Build history of the part. All positions in model axes, mm. A direction names the side the tool comes from. Give positions to 0.01 mm unless a question says otherwise; leave off trailing zeros. Loops run counter-clockwise (first coordinate to the right, second up) from the corner with the lowest first, then second, coordinate; pieces in that order, holes last. Notation, with made-up numbers: (40.5, 79) -> (82.5, 79) arc R24 ccw to (82.5, 97) -> close; hole circle Ø8 at (-6.75, -26). An arc over 180 degrees is marked (long way). Answer as a JSON object with one key per item and string values. Group by question number.
Q1. Band-saw the part on A-A, the plane y = 6. Write the cut outline in (x, z) (1 decimal).
Q2. Wall check: probe 1 along X at (y, z) = (19, -53) (1 decimal); probe 2 along Y at (x, z) = (683.5, -31.5). Give the ranges that are in metal, low to high. Write a range as from..to.
Q3. Drop flat-ended pins along their axis: pin 1 (9.5 mm diameter, centred on y = 8, z = -32, fed in from -X); pin 2 (1.5 mm diameter, centred on x = 700.5, z = -28.5, fed in from -Y). Give the stop position or say it passes through.
Q4. Band-saw the part on C-C, the plane x = 724.5. Write the cut outline in (y, z), plus the area to 3 significant figures.
Q5. Two-plate mould, pull along X, no slides. Class faces 1 (the flat face through (738.188, 9, -44)), 2 (the flat face through (790.575, 19, -44)), 3 (the flat face through (392, 0, -45)): pulls with the +X half, pulls with the -X half, needs draft (parallel to the pull), parting line crosses it, or undercut.
Q6. Tool access for faces 4 (the flat face through (96, 19.05, -44)), 5 (the flat face through (390, 38.1, -45)): list every direction of +Z, -Z, +X, -X, +Y, -Y with a clear straight run to the whole face (end or side of a thin tool).
from build123d import *

# Parameters (mm, degrees)
SKETCH1_W           = 790.575
SKETCH1_H           = 88.9
BOSS_EXTRUDE1_DEPTH = 38.1
SKETCH2_W           = 88.9
SKETCH2_H           = 19.05
CUT_EXTRUDE1_DEPTH  = 89.9


with BuildPart() as part:
    # Sketch1 → Boss-Extrude1 (new body)
    with BuildSketch(Plane(origin=(0, 0, 0), x_dir=(1, 0, 0), z_dir=(0, 1, 0))):
        with Locations((395.2875, 44.45)):
            Rectangle(SKETCH1_W, SKETCH1_H)
    extrude(amount=BOSS_EXTRUDE1_DEPTH)

    # Sketch2 → Cut-Extrude1 (cut, through all)
    with BuildSketch(Plane.XY):
        with Locations((693.7375, 9.525)):
            Rectangle(SKETCH2_W, SKETCH2_H)
        with Locations((96.8502, 9.525)):
            Rectangle(SKETCH2_W, SKETCH2_H)
    extrude(amount=-CUT_EXTRUDE1_DEPTH, mode=Mode.SUBTRACT)


solid = part.part
Worked answers:
{
 "1": {"outline": "(0, -88.9) -> (52.4, -88.9) -> (52.4, 0) -> (0, 0) -> close; (141.3, -88.9) -> (649.3, -88.9) -> (649.3, 0) -> (141.3, 0) -> close; (738.2, -88.9) -> (790.6, -88.9) -> (790.6, 0) -> (738.2, 0) -> close"},
 "2": {"probe 1": "0..52.4, 141.3..649.3, 738.2..790.6", "probe 2": "19.05..38.1"},
 "3": {"pin 1": "x = 0", "pin 2": "y = 19.05"},
 "4": {"outline": "(19.05, -88.9) -> (38.1, -88.9) -> (38.1, 0) -> (19.05, 0) -> close", "area": "1,690 mm2"},
 "5": {"face 1": "undercut", "face 2": "pulls with the +X half", "face 3": "needs draft"},
 "6": {"face 4": "+Z, -Z, -Y", "face 5": "+Z, -Z, +X, -X, +Y"}
}
